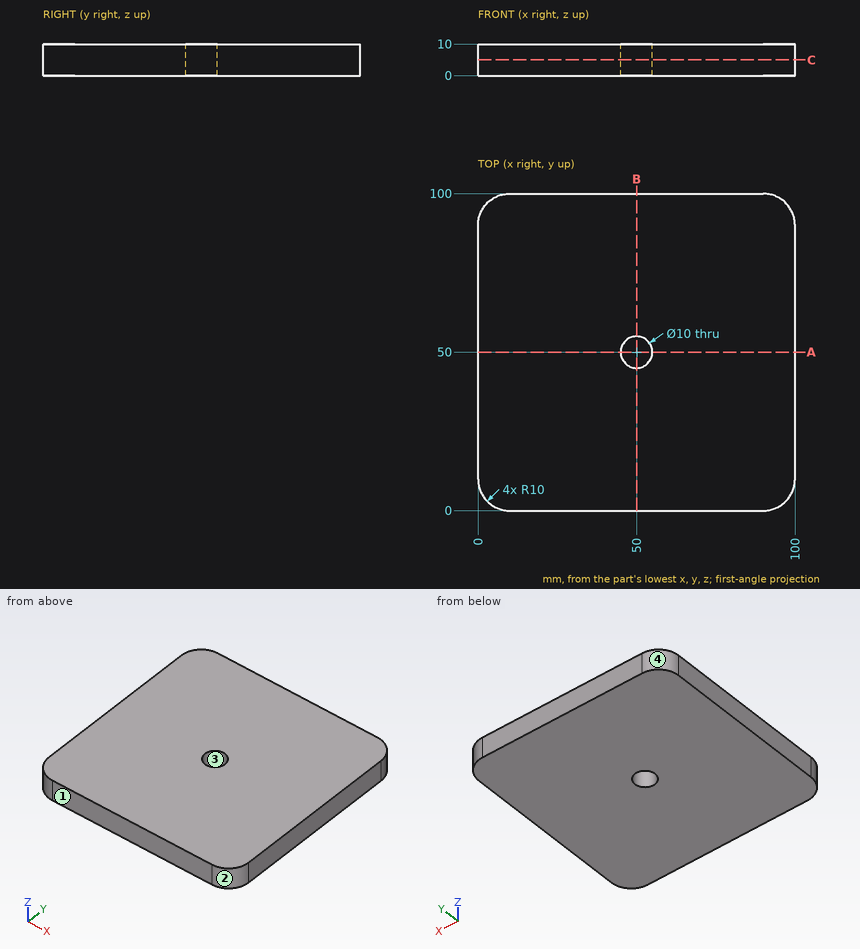
Could you check a few things on this drawing? It's one solid part, dimensions in mm from its lowest x, y, z. Round coordinates to 2 decimals unless told otherwise and drop trailing zeros. Loops run counter-clockwise (first coordinate to the right, second up) from the corner with the lowest first, then second, coordinate; pieces in that order, holes last. Notation, with made-up numbers: M -21.5,-23 L 28.5,-23 A21 cw 28.5,-7 Z; hole C -34,45 d4. An arc over 180 degrees is marked long. Write item = value, one per line. Start each with the question number.
(1) Suppose I cut it at C-C on z = 5. Write out the boundary of the cut face in (x, y).
(2) If we mould it in two halves opening along X, with no side actions, what happens to the marked faces 1, 2, 3 and 4? For each: released by +X, released by -X, zero draft, split by the parting line, or undercut.
(3) I'm going to push flat-ended pins straight in: P1, Ø6, axis at x = 83.5, z = 2.5, coming from the -Y side; P2, Ø9, axis at x = 50, y = 50, coming from the +Z side. Where does each tip first touch, or does it pass through?
(4) Suppose I cut it at A-A on y = 50. Write out the boundary of the cut face in (x, z), plus the area to 3 significant figures.
(5) I need wall thicknesses on line 1 along Y through (x, z) = (50, 2); line 2 along Y through (x, z) = (4, 7). Which ranges of each line are inside material? Lowest first, please.
Answer block:
q1.outline = M 0,10 A10 ccw 10,0 L 90,0 A10 ccw 100,10 L 100,90 A10 ccw 90,100 L 10,100 A10 ccw 0,90 Z; hole C 50,50 d10
q2.face_1 = zero draft
q2.face_2 = released by +X
q2.face_3 = undercut
q2.face_4 = released by -X
q3.P1 = 0
q3.P2 = through
q4.outline = M 0,0 L 45,0 L 45,10 L 0,10 Z; M 55,0 L 100,0 L 100,10 L 55,10 Z
q4.area = 900 mm²
q5.line_1 = 0 to 45, 55 to 100
q5.line_2 = 2 to 98
